```python
from build123d import *

# Parameters (mm, degrees)
F0_W     = 20.3
F0_H     = 5
F0_W_2   = 10.6
F0_H_2   = 2.05
F1_DEPTH = 6.25
F2_R     = 0.75
F3_DEPTH = 3.9


with BuildPart() as f1:
    # F0 (on Top) → F1 (new body)
    with BuildSketch(Plane.XY):
        Rectangle(F0_W, F0_H)
        Rectangle(F0_W_2, F0_H_2, mode=Mode.SUBTRACT)
    extrude(amount=F1_DEPTH)

    # F2 (on Front) → F3 (cut, symmetric)
    with BuildSketch(Plane.XZ):
        with Locations((-7.65, 3.125)):
            Circle(F2_R)
        with Locations((7.65, 3.125)):
            Circle(F2_R)
    extrude(amount=F3_DEPTH, both=True, mode=Mode.SUBTRACT)


solid = f1.part
```
Verification items for the finished model (mm, model axes). A direction names the side the tool comes from. Coordinates: 2 decimals unless noted, no trailing zeros. Write each loop counter-clockwise with the first axis right and the second up, starting at its lowest first coordinate (ties: lowest second). Pieces come first, ordered by that corner, then holes. Notation, with made-up numbers: M 43,60.25 L 67,60.25 A17 ccw 67,89.25 Z; hole C 22,81.25 d3. An arc over 180 degrees is marked long. One line per item, written item: value.
Item 1: Access from +Z, -Z, +X, -X, +Y, -Y to the whole of each face (thin tool, end or side, straight path). Record for faces 1 (the flat face through (0, 2, 6.25)), 2 (the flat face through (0, 1.025, 3)).
Check sheet entries:
face 1: +Z, +X, -X, +Y, -Y
face 2: +Z, -Z
Item 2: Section check C-C, the plane z = 4.25. Record the boundary of the cut face in (x, y) (3 decimals), plus the area to 3 significant figures.
Check sheet entries:
outline: M -10.15,-2.5 L 10.15,-2.5 L 10.15,2.5 L -10.15,2.5 Z; hole M -5.3,-1.025 L 5.3,-1.025 L 5.3,1.025 L -5.3,1.025 Z
area: 79.8 mm^2
Item 3: Section check A-A, the plane x = 0.5. Record the boundary of the cut face in (y, z) (3 decimals).
Check sheet entries:
outline: M -2.5,0 L -1.025,0 L -1.025,6.25 L -2.5,6.25 Z; M 1.025,0 L 2.5,0 L 2.5,6.25 L 1.025,6.25 Z
Item 4: Section check D-D, the plane x = -7.65. Record the boundary of the cut face in (y, z) (3 decimals), plus the area to 4 significant figures.
Check sheet entries:
outline: M -2.5,0 L 2.5,0 L 2.5,2.375 L -2.5,2.375 Z; M -2.5,3.875 L 2.5,3.875 L 2.5,6.25 L -2.5,6.25 Z
area: 23.75 mm^2
Item 5: Mould release check, pull along Y, two halves, no side actions. Record for faces 3 (the flat face through (-5.3, 0, 3)), 4 (the flat face through (0, -2.5, 3)), 5 (the flat face through (0, 2.5, 3)), 6 (the flat face through (-10.15, 0, 3)): pulls with the +Y half, pulls with the -Y half, needs draft (parallel to the pull), parting line crosses it, or undercut.
Check sheet entries:
face 3: undercut
face 4: pulls with the -Y half
face 5: pulls with the +Y half
face 6: needs draft
Item 6: Section check B-B, the plane y = 0.4. Record the boundary of the cut face in (x, z) (3 decimals), plus the area to 3 significant figures.
Check sheet entries:
outline: M -10.15,0 L -5.3,0 L -5.3,6.25 L -10.15,6.25 Z; M 5.3,0 L 10.15,0 L 10.15,6.25 L 5.3,6.25 Z; hole C -7.65,3.125 d1.5; hole C 7.65,3.125 d1.5
area: 57.1 mm^2
Item 7: Scan lines: line 1 along Y through (x, z) = (4.5, 3.75) (3 decimals); line 2 along X through (y, z) = (0.9, 1.5); line 3 along Z through (x, y) = (7.65, -0.6) (3 decimals). Record each from-to range of solid material in increasing order.
Check sheet entries:
line 1: y = -2.5 to -1.025, 1.025 to 2.5
line 2: x = -10.15 to -5.3, 5.3 to 10.15
line 3: z = 0 to 2.375, 3.875 to 6.25
